from build123d import *

# Parameters (mm, degrees)
BOSS_EXTRUDE1_DEPTH = 14
SKETCH2_R           = 2.25
CUT_EXTRUDE1_DEPTH  = 42.328712779
SKETCH4_W           = 47.5
SKETCH4_H           = 13
CUT_EXTRUDE3_DEPTH  = 42.328712779
CHAMFER1_SIZE       = 6.92820323
CHAMFER1_SIZE_2     = 4
CHAMFER2_SIZE       = 3.8
CHAMFER2_SIZE2      = 6.581793069


with BuildPart() as part:
    # Sketch1 → Boss-Extrude1 (new, symmetric)
    with BuildSketch(Plane(origin=(0, 0, 0), x_dir=(1, 0, 0), z_dir=(0, 1, 0))):
        Polygon((-5, -20.25), (-5, 23.25), (-7, 23.25), (-7, 38.25), (0, 38.25), (0, -38.25), (-5, -38.25), (-5, -28.25), (-6, -28.25), (-6, -20.25), align=None)
    extrude(amount=BOSS_EXTRUDE1_DEPTH, both=True)

    # Sketch2 → Cut-Extrude1 (cut, through all)
    with BuildSketch(Plane(origin=(0, 0, 0), x_dir=(0, 0, -1), z_dir=(1, 0, 0))):
        with Locations((-24.25, -4)):
            Circle(SKETCH2_R)
    extrude(amount=-CUT_EXTRUDE1_DEPTH, mode=Mode.SUBTRACT)

    # Sketch4 → Cut-Extrude3 (cut, through all)
    with BuildSketch(Plane(origin=(0, 0, 0), x_dir=(0, 0, -1), z_dir=(1, 0, 0))):
        with Locations((14.5, 7.5)):
            Rectangle(SKETCH4_W, SKETCH4_H)
    extrude(amount=-CUT_EXTRUDE3_DEPTH, mode=Mode.SUBTRACT)

    # Chamfer1
    # the kernel refuses this chamfer: 6.92820323, 4 mm, written as the material it takes off along each edge
    with BuildSketch(Plane(origin=(0, 14, -8.673855882), x_dir=(-0.9998132206222079, 0.01932676561270069, 0), z_dir=(0, 0, 1))) as chamfer1_piece_1:
        Polygon((CHAMFER1_SIZE * 0.999813220662, CHAMFER1_SIZE * 0.0193267656135), (-CHAMFER1_SIZE_2 * 0.0193267656127, CHAMFER1_SIZE_2 * 0.999813220622), (0, 0), align=None)
    extrude(amount=64.847711765, mode=Mode.SUBTRACT)

    # Chamfer2
    chamfer2_edges = [part.edges().sort_by_distance(p)[0] for p in [
        (0, 1, -14.5),
    ]]
    chamfer2_side = [part.faces().sort_by_distance(p)[0] for p in [
        (0, -4.279514007, 4.174270011),
    ]]
    chamfer(chamfer2_edges, length=CHAMFER2_SIZE, length2=CHAMFER2_SIZE2, reference=chamfer2_side[0])


solid = part.part
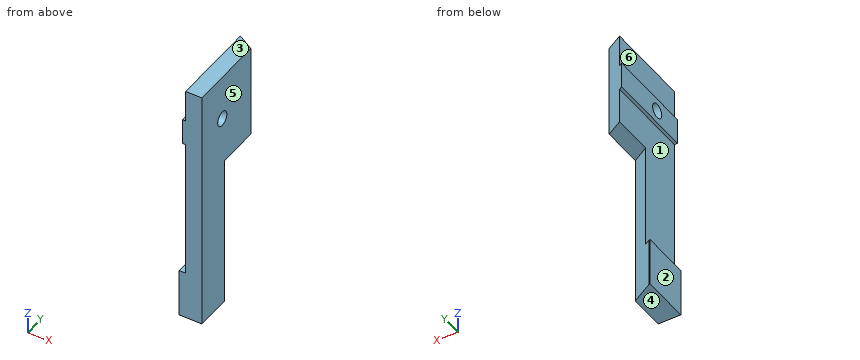
Work out the finished part from the listing and answer in its coordinate system (mm). Face numbers are marked on the shaded views. A direction names the side the tool comes from. Round coordinates to 2 decimals unless told otherwise and drop trailing zeros. Write each loop counter-clockwise with the first axis right and the second up, starting at its lowest first coordinate (ties: lowest second). Pieces come first, ordered by that corner, then holes.
1) A cutting plane is placed at B-B (y = -4). Give the vertices of the cut face in (x, z).
2) A tool of negligible diameter and unlimited length cuts with its end or side. For the marked faces 5 and 6, from which of +Z, -Z, +X, -X, +Y, -Y can it reach the whole face along a straight path? Write none if from no direction.
3) A cutting plane is placed at A-A (z = 24.25). Give the vertices of the cut face in (x, y), plus the area to 3 significant figures.
4) Given pin 1 Ø6 at (y, z) = (4.5, -0.5) entering from -X; pin 2 Ø4 at (y, z) = (0, 23) entering from -X; pin 3 Ø13.5 at (y, z) = (-6.5, -9.5) entering from -X; pin 4 Ø2.5 at (x, y) = (-2.5, 3) entering from -Z, each flat-ended and moving along its own axis, determine where each tip first touches the part or whether it passes through.
5) The mould has two halves that part along Z. Classify the marked faces 1, 2, 3 and 4: pulls with the +Z half, pulls with the -Z half, needs draft (parallel to the pull), parting line crosses it, or undercut.
6) Straight lines are drawn through the part: line 1 (X direction, y = -8.5, z = 19.5); line 2 (Y direction, x = -3.95, z = 24.25); line 3 (Y direction, x = -1.15, z = 24.25). For each, find the intervals that lie inside material, in ascending order.
7) A cutting plane is placed at C-C (x = -4). Give the vertices of the cut face in (y, z).
8) A cutting plane is placed at D-D (y = 4.5). Give the vertices of the cut face in (x, z).
Completed:
1. outline: (-7, -38.25) - (0, -38.25) - (0, 22) - (-6, 22) - (-6, 20.25) - (-5, 20.25) - (-5, -23.25) - (-7, -23.25) - close; (-6, 26.5) - (0, 26.5) - (0, 38.25) - (-5, 38.25) - (-5, 28.25) - (-6, 28.25) - close
2. face 5: +Z, -Z, +X, +Y, -Y
2. face 6: +Z, -X, +Y, -Y
3. outline: (-6, -14) - (0, -14) - (0, -6.25) - (-6, -6.25) - close; (-6, -1.75) - (0, -1.75) - (0, 10) - (-6, 13.46) - close
3. area: 127 mm2
4. pin 1: passes through
4. pin 2: stops at x = -6
4. pin 3: stops at x = -5
4. pin 4: stops at z = 9.25
5. face 1: undercut
5. face 2: needs draft
5. face 3: pulls with the +Z half
5. face 4: pulls with the -Z half
6. line 1: x = -5 to 0
6. line 2: y = -14 to -6.25, -1.75 to 12.28
6. line 3: y = -14 to -6.25, -1.75 to 10.66
7. outline: (-14, -38.25) - (-0.49, -38.25) - (-0.49, 9.25) - (12.31, 9.25) - (12.31, 38.25) - (-14, 38.25) - close; hole circle Ø4.5 at (-4, 24.25)
8. outline: (-6, 20.25) - (-5, 20.25) - (-5, 9.25) - (0, 9.25) - (0, 38.25) - (-5, 38.25) - (-5, 28.25) - (-6, 28.25) - close
